from build123d import *

# Parameters (mm, degrees)
SKETCH_1_R                       = 1.15
EXTRUDE_1_DEPTH                  = 4
FILLET_1_R                       = 2
FILLET_2_R                       = 1
REVOLVE_2_ANGLE                  = 83
PATTERN_CIRCULAR_4_COUNT         = 2
PATTERN_CIRCULAR_4_ANGLE         = 83
FILLET_1_OF_PATTERN_CIRCULAR_4_R = 2
FILLET_2_OF_PATTERN_CIRCULAR_4_R = 1


with BuildPart() as part:
    # 草图1 → 凸台-拉伸1 (new body)
    with BuildSketch(Plane(origin=(0, 0, 0), x_dir=(1, 0, 0), z_dir=(0, 1, 0))):
        with BuildLine():
            Line((15, 20), (25, 30))
            Line((25, 30), (25, 40))
            Line((25, 40), (30, 45))
            Line((30, 45), (30, 65))
            Line((30, 65), (36, 65))
            Line((36, 65), (36, 43.100505063))
            Line((36, 43.100505063), (30.563454525, 37.663959588))
            Line((30.563454525, 37.663959588), (30.563454525, 25.663959588))
            Line((30.563454525, 25.663959588), (19.956852807, 15.05735787))
            ThreePointArc((19.956852807, 15.05735787), (17.652275132, 17.7030275), (15, 20))
        make_face()
        with Locations(Location((33, 60, 0), (0, 0, 270))):
            Circle(SKETCH_1_R, mode=Mode.SUBTRACT)
        with Locations(Location((33, 52, 0), (0, 0, 270))):
            Circle(SKETCH_1_R, mode=Mode.SUBTRACT)
    extrude_1 = extrude(amount=EXTRUDE_1_DEPTH)

    # 圆角1
    fillet_1_edges = [part.edges().sort_by_distance(p)[0] for p in [
        (30, 2, -45),
        (30, 2, -65),
        (36, 2, -65),
        (36, 2, -43.100505063),
        (30.563454525, 2, -37.663959588),
        (30.563454525, 2, -25.663959588),
    ]]
    fillet(fillet_1_edges, radius=FILLET_1_R)

    # 圆角2
    fillet_2_edges = [part.edges().sort_by_distance(p)[0] for p in [
        (19.956852807, 2, -15.05735787),
    ]]
    fillet(fillet_2_edges, radius=FILLET_2_R)

    # 草图2 → 旋转2 (revolve)
    with BuildSketch(Plane(origin=(0, 2, 0), x_dir=(1, 0, 0), z_dir=(0, 1, 0))):
        with BuildLine():
            Line((28.563454525, 26.492386713), (28.563454525, 36.835532463))
            Line((28.563454525, 36.835532463), (25, 36.835532463))
            Line((25, 36.835532463), (25, 30))
            Line((25, 30), (15, 20))
            ThreePointArc((15, 20), (16.926416038, 18.398272748), (18.682847286, 16.611779474))
            Line((18.682847286, 16.611779474), (28.563454525, 26.492386713))
        make_face()
    revolve(axis=Axis((0, 2, -67.472032035), (0, 0, 1)), revolution_arc=REVOLVE_2_ANGLE)

    # 阵列(圆周)4: 凸台-拉伸1 ×2 about axis
    pattern_circular_4_axis = Axis((0, 2, 0), (0, 0, 1))
    for i in range(1, PATTERN_CIRCULAR_4_COUNT):
        add(extrude_1.rotate(pattern_circular_4_axis, i * PATTERN_CIRCULAR_4_ANGLE / (PATTERN_CIRCULAR_4_COUNT - 1)))

    # 圆角1 of 阵列(圆周)4
    fillet_1_of_pattern_circular_4_edges = [part.edges().sort_by_distance(p)[0] for p in [
        (3.656080302, 31.776384549, -45),
        (3.656080302, 31.776384549, -65),
        (4.387296363, 37.731661459, -65),
        (4.387296363, 37.731661459, -43.100505063),
        (3.724748135, 32.335639169, -37.663959588),
        (3.724748135, 32.335639169, -25.663959588),
    ]]
    fillet(fillet_1_of_pattern_circular_4_edges, radius=FILLET_1_OF_PATTERN_CIRCULAR_4_R)

    # 圆角2 of 阵列(圆周)4
    fillet_2_of_pattern_circular_4_edges = [part.edges().sort_by_distance(p)[0] for p in [
        (2.432128548, 21.808097452, -15.05735787),
    ]]
    fillet(fillet_2_of_pattern_circular_4_edges, radius=FILLET_2_OF_PATTERN_CIRCULAR_4_R)


solid = part.part
Geometry: final body of the model. Coordinates: model frame, mm. A direction names the side the tool comes from. Round coordinates to 2 decimals unless told otherwise and drop trailing zeros. Order: outer loops, then holes, each group sorted by start corner. A loop starts at its lowest first (then second) coordinate and runs counter-clockwise, first axis right, second up.
Q1. Section C-C, the plane z = -35. Output: boundary loops of the cut face in (x, y), and give its area (3 significant figures).
Result sheet:
outline: (1.06, 27.06) - (3.05, 26.81) arc R25 cw to (25, 2) - (25, 0) - (30.56, 0) - (30.56, 4) - (28.49, 4) arc R28.56 ccw to (5.46, 30.04) - (5.71, 32.09) - (1.74, 32.58) - close
area: 169 mm2
Q2. Pin query (flat end, axial travel): pin 1 (1.2 mm diameter, centred on y = 2, z = -36, fed in from -X); pin 2 (1.5 mm diameter, centred on x = 20.5, z = -32, fed in from +Y); pin 3 (4.5 mm diameter, centred on y = 1, z = -55, fed in from -X); pin 4 (1.4 mm diameter, centred on x = 33, z = -60, fed in from +Y). Return the tip coordinate at first contact, or that it passes through.
Result sheet:
pin 1: stops at x = 24.99
pin 2: stops at y = 22.64
pin 3: stops at x = 30
pin 4: passes through
Q3. Section A-A, the plane z = -49. Output: boundary loops of the cut face in (x, y), and give its area (3 significant figures).
Result sheet:
outline: (1.67, 32.02) - (5.64, 31.53) - (6.37, 37.49) - (2.4, 37.98) - close; (30, 0) - (36, 0) - (36, 4) - (30, 4) - close
area: 48.0 mm2
Q4. Section B-B, the plane x = 33. Output: boundary loops of the cut face in (y, z).
Result sheet:
outline: (0, -65) - (4, -65) - (4, -61.15) - (0, -61.15) - close; (0, -58.85) - (4, -58.85) - (4, -53.15) - (0, -53.15) - close; (0, -50.85) - (4, -50.85) - (4, -40.1) - (0, -40.1) - close
Q5. Mould query, pull axis Y, two halves, no side actions, for faces 4 (the face through (25.4, 2, -20.5)), 5 (the face through (31, 4, -44)), 6 (the face through (4.09, 35.09, -58.9)). Classes: released by +Y, released by -Y, zero draft, split by the parting line, or undercut.
Result sheet:
face 4: zero draft
face 5: released by +Y
face 6: undercut
Q6. Section D-D, the plane z = -23.5. Output: boundary loops of the cut face in (x, y).
Result sheet:
outline: (0.27, 20.61) - (2.25, 20.36) arc R18.5 cw to (18.5, 2) - (18.5, 0) - (28.4, 0) - (28.4, 4) - (25.49, 4) arc R25.57 ccw to (5.09, 27.06) - (5.45, 29.94) - (1.48, 30.43) - close
Q7. Material intervals for probe 1 along X at (y, z) = (2.95, -60); probe 2 along Y at (x, z) = (28, -38); probe 3 along Y at (x, z) = (4, -51), sorted ascending.
Result sheet:
probe 1: x = 30 to 31.85, 34.15 to 36
probe 2: y = 0 to 4
probe 3: y = 31.73 to 34.18, 35.33 to 37.78
Q8. Access query for faces 1 (the face through (1.413, 29.918, -38.564)), 2 (the face through (3.684, 31.773, -54.294)), 3 (the face through (30.563, 2, -32)). Directions: +Z, -Z, +X, -X, +Y, -Y. A direction counts if a zero-diameter tool reaches every point of the face in a straight line with its end or side. Return the directions, or none.
Result sheet:
face 1: +Z, -Z, -X, +Y
face 2: -Z, -X, -Y
face 3: +Z, +X, +Y, -Y
